The model under review builds one solid part; all positions refer to its coordinate system, in mm. A direction names the side the tool comes from. Round coordinates to 2 decimals unless told otherwise and drop trailing zeros. Write each loop counter-clockwise with the first axis right and the second up, starting at its lowest first coordinate (ties: lowest second). Pieces come first, ordered by that corner, then holes.
Item 1: Add section A-A (x = 10). Give the boundary of the cut face in (y, z), plus the area to 3 significant figures.
Item 2: Add section C-C (y = 17.5). Give the boundary of the cut face in (x, z).
Item 3: Add section D-D (z = -10). Give the boundary of the cut face in (x, y).
Item 4: Clearance check with flat-ended pins moving along their axes: pin 1 Ø1.5 at (y, z) = (19.5, -17) entering from +X; pin 2 Ø10 at (y, z) = (34, -13) entering from -X; pin 3 Ø2 at (x, z) = (45, -11.5) entering from -Y. State where each tip first meets the part, or that it passes through.
Item 5: Machinability: for faces 1 (the face through (44, 24.5, -10)), 2 (the face through (0, 33, -10)), 3 (the face through (14.212, 39.472, -14.594)), 4 (the face through (0, 12, -10)), 5 (the face through (44, 28.5, -10)), which of the approach directions +Z, -Z, +X, -X, +Y, -Y give a long, thin tool a straight path to every point of the face, cutting with its end or side? Answer none if there is none.
Item 6: To check wall thickness, follow L1, parallel to X at y = 38.6, z = -10; L2, parallel to Y at x = 36.5, z = -9.25; L3, parallel to X at y = 36, z = -2.5. State the ranges of each line that lie inside material, in increasing order.
Item 7: Draft analysis for pull direction Z (two halves, no side actions). For faces 6 (the face through (40, 12, -10)), 7 (the face through (12.7, 39.47, -12.95)), 8 (the face through (20, 18, 0)), 9 (the face through (20, 18, -20)), state which applies: +Z half, -Z half, draft (parallel to the pull), parting line (faces both ways), or undercut.
Item 8: Add section B-B (z = -2.75). Give the boundary of the cut face in (x, y).
```python
from build123d import *

# Parameters (mm, degrees)
SKETCH1_W           = 40
SKETCH1_H           = 20
BOSS_EXTRUDE1_DEPTH = 24.5
SKETCH2_W           = 54.5
SKETCH2_H           = 20
BOSS_EXTRUDE2_DEPTH = 4
SKETCH3_W           = 40
SKETCH3_H           = 37.5
BOSS_EXTRUDE3_DEPTH = 20
SKETCH8_R           = 6.232527985
SKETCH8_R_2         = 4
BOSS_EXTRUDE4_DEPTH = 4


with BuildPart() as part:
    # Sketch1 → Boss-Extrude1 (new body)
    with BuildSketch(Plane(origin=(0, 0, 0), x_dir=(1, 0, 0), z_dir=(0, 1, 0))):
        with Locations((20, 10)):
            Rectangle(SKETCH1_W, SKETCH1_H)
    extrude(amount=BOSS_EXTRUDE1_DEPTH)

    # Sketch2 → Boss-Extrude2 (add)
    with BuildSketch(Plane(origin=(0, 24.5, 0), x_dir=(1, 0, 0), z_dir=(0, 1, 0))):
        with Locations((20, 10)):
            Rectangle(SKETCH2_W, SKETCH2_H)
    extrude(amount=BOSS_EXTRUDE2_DEPTH)

    # Sketch3 → Boss-Extrude3 (add)
    with BuildSketch(Plane.XY):
        with Locations((20, 18.75)):
            Rectangle(SKETCH3_W, SKETCH3_H)
    extrude(amount=-BOSS_EXTRUDE3_DEPTH)

    # Sketch8 → Boss-Extrude4 (add)
    with BuildSketch(Plane(origin=(0, 37.5, 0), x_dir=(1, 0, 0), z_dir=(0, 1, 0))):
        with Locations(Location((10, 10, 0), (0, 0, 270))):
            Circle(SKETCH8_R)
        with Locations(Location((10, 10, 0), (0, 0, 270))):
            Circle(SKETCH8_R_2, mode=Mode.SUBTRACT)
    extrude(amount=BOSS_EXTRUDE4_DEPTH)


solid = part.part
```
Numbers:
1. outline: (0, -20) - (37.5, -20) - (37.5, -16.23) - (41.5, -16.23) - (41.5, -14) - (37.5, -14) - (37.5, -6) - (41.5, -6) - (41.5, -3.77) - (37.5, -3.77) - (37.5, 0) - (0, 0) - close
1. area: 768 mm2
2. outline: (0, -20) - (40, -20) - (40, 0) - (0, 0) - close
3. outline: (-7.25, 24.5) - (0, 24.5) - (0, 0) - (40, 0) - (40, 24.5) - (47.25, 24.5) - (47.25, 28.5) - (40, 28.5) - (40, 37.5) - (16.23, 37.5) - (16.23, 41.5) - (14, 41.5) - (14, 37.5) - (6, 37.5) - (6, 41.5) - (3.77, 41.5) - (3.77, 37.5) - (0, 37.5) - (0, 28.5) - (-7.25, 28.5) - close
4. pin 1: stops at x = 40
4. pin 2: stops at x = 0
4. pin 3: stops at y = 24.5
5. face 1: +Z, -Z, +X, -Y
5. face 2: +Z, -Z, -X, +Y
5. face 3: +Y
5. face 4: +Z, -Z, -X, -Y
5. face 5: +Z, -Z, +X, +Y
6. L1: x = 3.77 to 6, 14 to 16.23
6. L2: y = 0 to 37.5
6. L3: x = 0 to 40
7. face 6: draft
7. face 7: undercut
7. face 8: +Z half
7. face 9: -Z half
8. outline: (-7.25, 24.5) - (0, 24.5) - (0, 0) - (40, 0) - (40, 24.5) - (47.25, 24.5) - (47.25, 28.5) - (40, 28.5) - (40, 37.5) - (0, 37.5) - (0, 28.5) - (-7.25, 28.5) - close
